Verification items for the finished model (mm, model axes). A direction names the side the tool comes from. Coordinates: 2 decimals unless noted, no trailing zeros. Order: outer loops, then holes, each group sorted by start corner. A loop starts at its lowest first (then second) coordinate and runs counter-clockwise, first axis right, second up. Notation, with made-up numbers: M -36.75,78 L -17.75,78 A16 ccw -17.75,103 Z; hole C 89,-29.75 d11. An arc over 180 degrees is marked long. Write item = value, one per line.
Autodesk Inventor part; units mm, degrees
ref_plane "Startebene" through (0, 0, 0) normal (1, 0, 0) x (0, 1, 0)
ref_plane "XZ Plane" through (0, 0, 0) normal (0, 1, 0) x (-1, 0, 0)
ref_plane "XY Plane" through (0, 0, 0) normal (0, 0, 1) x (1, 0, 0)
sketch "Hauptskizze" plane through (0, 0, 0) normal (0, 0, 1) x (1, 0, 0)
  line L0 (0, 0) -> (25, 0)
  line L1 (0, 0) -> (0, 2.5)
  line L2 (0, 2.5) -> (5, 2.5)
  line L3 (5, 2.5) -> (5, 4)
  line L4 (6, 4) -> (6, 3.5)
  line L5 (5, 4) -> (6, 4)
  line L6 (6, 3.5) -> (19, 3.5)
  line L7 (20, 4) -> (20, 2.5)
  line L8 (19, 4) -> (20, 4)
  line L9 (25, 2.5) -> (25, 0)
  line L10 (20, 2.5) -> (25, 2.5)
  line L11 (19, 3.5) -> (19, 4)
  dimension "d3" = 5
  dimension "d4" = 8
  dimension "d5" = 7
  dimension "d13" = 8
  dimension "d14" = 5
revolve "Umdrehung1" add sketch "Hauptskizze" angle 360 about axis through (0, 0, 0) along (1, 0, 0)
chamfer "Fase5" distance 0.5 angle 45 1 edges at (19, -4, 0) measured on face at (19.3333, 3.987, -0.3219)
chamfer "Fase4" distance 0.5 angle 45 1 edges at (6, -4, 0) measured on face at (5.3333, 3.987, -0.3219)
chamfer "Fase3" distance 0.5 angle 45 1 edges at (25, -2.5, 0) measured on face at (21.6667, 2.4676, -0.401)
chamfer "Fase1" distance 0.5 angle 45 1 edges at (0, -2.5, 0) measured on face at (1.6667, 2.4676, -0.401)
properties part number "Welle 5x4+6x15+5x4" material "Messing, weicher Gelbton"
Item 1: Sectioned sample at C-C, the plane x = 4.75. Enter the section's corners in (y, z).
Report:
outline = C 0,0 d5
Item 2: Sectioned sample at D-D, the plane x = 18.25. Enter the section's corners in (y, z).
Report:
outline = C 0,0 d7
Item 3: Gauge pin test, flat end, axial feed: pin 1 (3 mm diameter, centred on x = 15, y = 2.5, fed in from +Z). Record the tip position at first contact, or that the pin passes through.
Report:
pin_1 = 3.35
Item 4: Scan lines: L1, parallel to X at y = -2.5, z = 2.25; L2, parallel to X at y = -3.5, z = -1; L3, parallel to X at y = -3, z = -2.5. Record each from-to range of solid material in increasing order. Write a range as from..to.
Report:
L1 = 5..20
L2 = 5..5.86, 19.14..20
L3 = 5..5.6, 19.4..20
Item 5: Tool access check on faces 4 (the flat face through (25, 0, 0)), 5 (the cylindrical face through (22.28, -0.54, -2.44)), 6 (the flat face through (5, 2, 2)). Record the directions out of +Z, -Z, +X, -X, +Y, -Y that give a thin tool (end or side, any length) a straight path to the whole face; none if there is none.
Report:
face_4 = +Z, -Z, +X, +Y, -Y
face_5 = +X
face_6 = -X
Item 6: Release check for a two-part mould opening along X. For faces 1 (the cylindrical face through (12.591, 3.233, -1.341)), 2 (the cylindrical face through (2.78, -0.54, -2.44)), 3 (the flat face through (0, 0, 0)) record: pulls with the +X half, pulls with the -X half, needs draft (parallel to the pull), parting line crosses it, or undercut.
Report:
face_1 = undercut
face_2 = needs draft
face_3 = pulls with the -X half
